The model under review builds one solid part; all positions refer to its coordinate system, in mm. Face numbers are marked on the shaded views. Round coordinates to 2 decimals unless told otherwise and drop trailing zeros. Loops run counter-clockwise (first coordinate to the right, second up) from the corner with the lowest first, then second, coordinate; pieces in that order, holes last. Notation, with made-up numbers: M -15.5,30 L -11.5,30 A23 ccw -11.5,53 Z; hole C 20.25,73 d3. An arc over 180 degrees is marked long. One line per question, with ' | ' between items.
from build123d import *

# Parameters (mm, degrees)
F1_DEPTH = 9.9
F2_R     = 34.0204521672
F3_DEPTH = 9.9
F4_D     = 28.6
F5_D     = 32


with BuildPart() as f1:
    # F0 (on Top) → F1 (new body)
    with BuildSketch(Plane.XY):
        with BuildLine():
            Line((-11.9994940177, 34.8422084712), (-0.0575622945, 55.5758049985))
            Line((-0.0575622945, 55.5758049985), (11.9272931484, 34.8669904922))
            ThreePointArc((11.9272931484, 34.8669904922), (16.2473796766, 38.0646478249), (19.7447123991, 42.1459250585))
            ThreePointArc((19.7447123991, 42.1459250585), (22.8148755334, 48.5513230922), (23.8692377055, 55.5758049985))
            ThreePointArc((23.8692377055, 55.5758049985), (-6.8934905458, 78.5053022276), (-20.0782891833, 42.4738107578))
            ThreePointArc((-20.0782891833, 42.4738107578), (-16.4881199464, 38.1824576068), (-11.9994940177, 34.8422084712))
        make_face()
        with BuildLine():
            ThreePointArc((19.7447123991, 42.1459250585), (16.2473796766, 38.0646478249), (11.9272931484, 34.8669904922))
            Line((11.9272931484, 34.8669904922), (36.1831113199, -7.0450076633))
            ThreePointArc((36.1831113199, -7.0450076633), (40.9619383877, -4.9383860109), (46.084167971, -3.9196578694))
            Line((46.084167971, -3.9196578694), (19.7447123991, 42.1459250585))
        make_face()
        with BuildLine():
            Line((-36.1522240312, -7.0917910472), (-11.9994940177, 34.8422084712))
            ThreePointArc((-11.9994940177, 34.8422084712), (-16.4881199464, 38.1824576068), (-20.0782891833, 42.4738107578))
            Line((-20.0782891833, 42.4738107578), (-46.7444930565, -3.9351598474))
            ThreePointArc((-46.7444930565, -3.9351598474), (-41.2637040523, -4.8938560089), (-36.1522240312, -7.0917910472))
        make_face()
        with BuildLine():
            ThreePointArc((46.084167971, -3.9196578694), (40.9619383877, -4.9383860109), (36.1831113199, -7.0450076633))
            Line((36.1831113199, -7.0450076633), (48.1588401117, -27.7380520899))
            Line((48.1588401117, -27.7380520899), (24.2502735607, -27.7628152391))
            ThreePointArc((24.2502735607, -27.7628152391), (25.0126751704, -33.7276444175), (27.2392931133, -39.3135745888))
            ThreePointArc((27.2392931133, -39.3135745888), (54.1364448927, -50.8873157676), (72.0674194868, -27.7380520899))
            ThreePointArc((72.0674194868, -27.7380520899), (64.3146084961, -10.1138835806), (46.084167971, -3.9196578694))
        make_face()
        with BuildLine():
            Line((-48.1012778172, -27.8377529085), (-36.1522240312, -7.0917910472))
            ThreePointArc((-36.1522240312, -7.0917910472), (-41.2637040523, -4.8938560089), (-46.7444930565, -3.9351598474))
            ThreePointArc((-46.7444930565, -3.9351598474), (-69.0295446869, -39.464552372), (-27.0898443417, -39.3135745888))
            ThreePointArc((-27.0898443417, -39.3135745888), (-24.9041765549, -33.7596878084), (-24.1602080848, -27.8377529085))
            ThreePointArc((-24.1602080848, -27.8377529085), (-24.1602112952, -27.8253545065), (-24.1602209263, -27.8129561077))
            Line((-24.1602209263, -27.8129561077), (-48.1012778172, -27.8377529085))
        make_face()
        with BuildLine():
            ThreePointArc((27.2392931133, -39.3135745888), (25.0126751704, -33.7276444175), (24.2502735607, -27.7628152391))
            Line((24.2502735607, -27.7628152391), (-24.1602209263, -27.8129561077))
            ThreePointArc((-24.1602209263, -27.8129561077), (-24.1602112952, -27.8253545065), (-24.1602080848, -27.8377529085))
            ThreePointArc((-24.1602080848, -27.8377529085), (-24.9041765549, -33.7596878084), (-27.0898443417, -39.3135745888))
            Line((-27.0898443417, -39.3135745888), (27.2392931133, -39.3135745888))
        make_face()
    extrude(amount=F1_DEPTH)

    # F2 (on Top) → F3 (join)
    with BuildSketch(Plane.XY):
        Circle(F2_R)
    extrude(amount=F3_DEPTH)

    # F4 (through all)
    with Locations(Plane(origin=(0, 0, 0), x_dir=(1, 0, 0), z_dir=(0, 0, -1))):
        with Locations((-0.0575622945, -55.5758049985), (48.1588401117, 27.7380520899), (-48.1012778172, 27.8377529085)):
            Hole(F4_D / 2)

    # F5 (through all)
    with Locations(Plane(origin=(0, 0, 0), x_dir=(1, 0, 0), z_dir=(0, 0, -1))):
        with Locations((0, 0)):
            Hole(F5_D / 2)


solid = f1.part
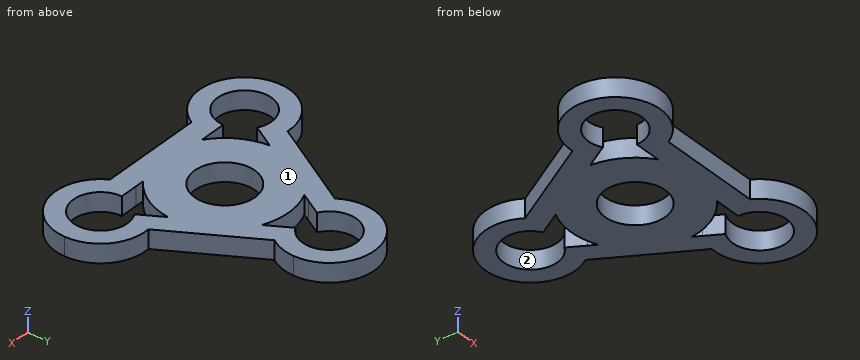
1) Add section A-A on x = 9.5. State the section outline as (y, z) points, then the cut area to 3 significant figures.
Output values:
outline: M -39.31,0 L -12.87,0 L -12.87,9.9 L -39.31,9.9 Z; M 12.87,0 L 32.67,0 L 32.67,9.9 L 12.87,9.9 Z; M 39.06,0 L 44.94,0 L 44.94,9.9 L 39.06,9.9 Z; M 66.21,0 L 77.51,0 L 77.51,9.9 L 66.21,9.9 Z | area: 628 mm²
2) For line 1 (X direction, y = -28.5, z = 1.5); line 2 (X direction, y = -9.5, z = 7.75); line 3 (Y direction, x = -8.5, z = 9.75), list the stretches that pass through material, from the lowest coordinate up.
Output values:
line 1: x = -72.03 to -62.39, -33.82 to 33.88, 62.44 to 72.06 | line 2: x = -63.49 to -37.54, -32.67 to -12.87, 12.87 to 32.67, 37.6 to 63.62 | line 3: y = -39.31 to -13.56, 13.56 to 32.94, 40.92 to 44.03, 67.12 to 77.96
3) Add section C-C on y = 0. State the section outline as (x, z) points, then the cut area to 3 significant figures.
Output values:
outline: M -44.48,0 L -16,0 L -16,9.9 L -44.48,9.9 Z; M 16,0 L 43.84,0 L 43.84,9.9 L 16,9.9 Z | area: 558 mm²
4) Add section D-D on y = 62.5. State the section outline as (x, z) points.
Output values:
outline: M -22.96,0 L -12.57,0 L -12.57,9.9 L -22.96,9.9 Z; M 12.45,0 L 22.85,0 L 22.85,9.9 L 12.45,9.9 Z
5) Insertion check: P1, Ø5, axis at x = 13.5, z = 6, coming from the -Y side; P2, Ø1.5, axis at x = -52.5, z = 1.5, coming from the +Y side; P3, Ø17, axis at x = 48.16, y = -27.74, coming from the -Z side; P4, Ø4, axis at y = -23.5, z = 2.5, coming from the -X side. Each pin has a flat end and moves straight along its axis. Give the tip position at first contact, or say it passes through.
Output values:
P1: stops at y = -39.31 | P2: stops at y = -4.18 | P3: passes through | P4: stops at x = -71.93
6) Mouldability with a two-part tool opening along X and no side actions: class the marked faces 1 and 2 as +X half, -X half, draft (parallel to the pull), parting line (faces both ways), or undercut.
Output values:
face 1: draft | face 2: undercut
7) Add section B-B on z = 7.25. State the section outline as (x, y) points (1 decimal), then the cut area to 3 significant figures.
Output values:
outline: M -46.7,-3.9 A23.9 ccw long -27.1,-39.3 L 27.2,-39.3 A23.9 ccw long 46.1,-3.9 L 19.7,42.1 A23.9 ccw long -20.1,42.5 Z; hole M -41,-15.4 A14.3 ccw long -33.8,-27.8 L -19.6,-27.8 A34 cw -33.9,-3.1 Z; hole C 0,0 d32; hole M -14.3,30.9 A34 cw 14.2,30.9 L 7.1,43.2 A14.3 ccw long -7.2,43.2 Z; hole M 19.7,-27.8 L 33.9,-27.8 A14.3 ccw long 41,-15.4 L 33.9,-3.1 A34 cw Z | area: 6,860 mm²
